```python
from build123d import *

# Parameters (mm, degrees)
SKETCH_1_R               = 2.05
SKETCH_1_R_2             = 1.05
SKETCH_1_R_3             = 1.55
SKETCH_1_R_4             = 1.25
EXTRUDE_1_DEPTH          = 4
EXTRUDE_START            = -4
EXTRUDE_2_DEPTH          = 6
SKETCH_4_R               = 1.05
CUT_EXTRUDE_2_DEPTH      = 11
SKETCH_5_R               = 1.2
CUT_EXTRUDE_3_DEPTH      = 114.5
FILLET_1_R               = 5
SKETCH_6_R               = 2.25
CUT_EXTRUDE_4_DEPTH      = 2.5
CHAMFER_1_SIZE           = 1.5
CUT_EXTRUDE_6_DEPTH      = 1
CUT_EXTRUDE_6_DEPTH_BACK = 11


with BuildPart() as part:
    # 草图1 → 凸台-拉伸1 (new body)
    with BuildSketch(Plane.XY):
        Polygon((20, -62), (5, -62), (5, -54.5), (-5, -54.5), (-5, -62), (-20, -62), (-20, 62), (-5, 62), (-5, 54.5), (5, 54.5), (5, 62), (20, 62), align=None)
        with Locations((10, 58.5)):
            Circle(SKETCH_1_R, mode=Mode.SUBTRACT)
        with Locations((-10, 58.5)):
            Circle(SKETCH_1_R, mode=Mode.SUBTRACT)
        with Locations((10, -58.5)):
            Circle(SKETCH_1_R, mode=Mode.SUBTRACT)
        with Locations((-10, -58.5)):
            Circle(SKETCH_1_R, mode=Mode.SUBTRACT)
        with Locations((-11, 6)):
            Circle(SKETCH_1_R_2, mode=Mode.SUBTRACT)
        with Locations((-11, -6)):
            Circle(SKETCH_1_R_2, mode=Mode.SUBTRACT)
        with Locations((11, -6)):
            Circle(SKETCH_1_R_2, mode=Mode.SUBTRACT)
        with Locations((11, 6)):
            Circle(SKETCH_1_R_2, mode=Mode.SUBTRACT)
        with Locations((-11.2, 0)):
            Circle(SKETCH_1_R_3, mode=Mode.SUBTRACT)
        with Locations((-14.35, -10)):
            Circle(SKETCH_1_R_4, mode=Mode.SUBTRACT)
        with Locations((-14.35, 10)):
            Circle(SKETCH_1_R_4, mode=Mode.SUBTRACT)
        with Locations((14.35, 10)):
            Circle(SKETCH_1_R_4, mode=Mode.SUBTRACT)
        with Locations((14.35, -10)):
            Circle(SKETCH_1_R_4, mode=Mode.SUBTRACT)
    extrude(amount=EXTRUDE_1_DEPTH)

    # 草图3 → 凸台-拉伸2 (add)
    with BuildSketch(Plane.XY.offset(4).offset(EXTRUDE_START)):
        Polygon((-20, 14.55), (20, 14.55), (20, 51.5), (14, 51.5), (14, 17.55), (-14, 17.55), (-14, 51.5), (-20, 51.5), align=None)
        Polygon((14, -17.55), (-14, -17.55), (-14, -51.5), (-20, -51.5), (-20, -14.55), (20, -14.55), (20, -51.5), (14, -51.5), align=None)
    extrude(amount=-EXTRUDE_2_DEPTH)

    # 草图4 → 切除-拉伸2 (cut, through all)
    with BuildSketch(Plane.XY.offset(4)):
        with Locations((-4.25753788, -55.24246212)):
            Circle(SKETCH_4_R)
        with Locations((4.25753788, -55.24246212)):
            Circle(SKETCH_4_R)
        with Locations((4.25753788, 55.24246212)):
            Circle(SKETCH_4_R)
        with Locations((-4.25753788, 55.24246212)):
            Circle(SKETCH_4_R)
    extrude(amount=-CUT_EXTRUDE_2_DEPTH, mode=Mode.SUBTRACT)

    # 草图5 → 切除-拉伸3 (cut, through all)
    with BuildSketch(Plane.XZ.offset(51.5)):
        with Locations((17, -3)):
            Circle(SKETCH_5_R)
        with Locations((-17, -3)):
            Circle(SKETCH_5_R)
    extrude(amount=-CUT_EXTRUDE_3_DEPTH, mode=Mode.SUBTRACT)

    # 圆角1
    fillet_1_edges = [part.edges().sort_by_distance(p)[0] for p in [
        (14, -17.55, -3),
        (-14, -17.55, -3),
        (-14, 17.55, -3),
        (14, 17.55, -3),
    ]]
    fillet(fillet_1_edges, radius=FILLET_1_R)

    # 草图6 → 切除-拉伸4 (cut)
    with BuildSketch(Plane.XY.offset(4)):
        with Locations((-11, -6)):
            Circle(SKETCH_6_R)
        with Locations((-11, 6)):
            Circle(SKETCH_6_R)
        with Locations((11, 6)):
            Circle(SKETCH_6_R)
        with Locations((11, -6)):
            Circle(SKETCH_6_R)
    extrude(amount=-CUT_EXTRUDE_4_DEPTH, mode=Mode.SUBTRACT)

    # 倒角1
    chamfer_1_edges = [part.edges().sort_by_distance(p)[0] for p in [
        (-12.75, 0, 4),
    ]]
    chamfer(chamfer_1_edges, length=CHAMFER_1_SIZE)

    # 草图8 → 切除-拉伸6 (cut, two sides)
    with BuildSketch(Plane.XY.offset(4)) as cut_extrude_6_sk:
        with BuildLine():
            Line((6, -17.55), (-6, -17.55))
            ThreePointArc((-6, -17.55), (-8.121320344, -18.428679656), (-9, -20.55))
            Line((-9, -20.55), (-9, -44.55))
            ThreePointArc((-9, -44.55), (-8.121320344, -46.671320344), (-6, -47.55))
            Line((-6, -47.55), (6, -47.55))
            ThreePointArc((6, -47.55), (8.121320344, -46.671320344), (9, -44.55))
            Line((9, -44.55), (9, -20.55))
            ThreePointArc((9, -20.55), (8.121320344, -18.428679656), (6, -17.55))
        make_face()
        with BuildLine():
            Line((-9, 20.55), (-9, 44.55))
            ThreePointArc((-9, 44.55), (-8.121320344, 46.671320344), (-6, 47.55))
            Line((-6, 47.55), (6, 47.55))
            ThreePointArc((6, 47.55), (8.121320344, 46.671320344), (9, 44.55))
            Line((9, 44.55), (9, 20.55))
            ThreePointArc((9, 20.55), (8.121320344, 18.428679656), (6, 17.55))
            Line((6, 17.55), (-6, 17.55))
            ThreePointArc((-6, 17.55), (-8.121320344, 18.428679656), (-9, 20.55))
        make_face()
    extrude(amount=CUT_EXTRUDE_6_DEPTH, mode=Mode.SUBTRACT)
    extrude(cut_extrude_6_sk.sketch, amount=-CUT_EXTRUDE_6_DEPTH_BACK, mode=Mode.SUBTRACT)


solid = part.part
```
For this review, take the finished solid that the model builds, in its own axes (mm). A direction names the side the tool comes from. Give positions to 0.01 mm unless a question says otherwise; leave off trailing zeros. Write each loop counter-clockwise with the first axis right and the second up, starting at its lowest first coordinate (ties: lowest second). Pieces come first, ordered by that corner, then holes.
Item 1: Take a section at D-D (z = -3). Give the number of separate pieces and of enclosed holes in the cut face, and give its area (3 significant figures).
Item 2: Take a section at B-B (y = -10). Give the boundary of the cut face in (x, z).
Item 3: Take a section at C-C (x = 17). Give the boundary of the cut face in (y, z), and give its area (3 significant figures).
Item 4: Insertion check: P1, Ø4.5, axis at x = 1.5, z = 3, coming from the -Y side; P2, Ø20, axis at x = 3.5, y = 29.5, coming from the -Z side; P3, Ø2.5, axis at x = -11, y = 6, coming from the +Z side. Each pin has a flat end and moves straight along its axis. Give the tip position at first contact, or say it passes through.
Item 5: Take a section at A-A (y = -35.5). Give the boundary of the cut face in (x, z).
Item 6: The part is to be moulded in two halves that separate along X. For faces 5 (the face through (14, -37, -3)), 6 (the face through (0, 0, 0)), say which applies: +X half, -X half, draft (parallel to the pull), parting line (faces both ways), or undercut.
Item 7: Machinability: for faces 1 (the face through (-12.5, 18.98, -3.04)), 2 (the face through (-5, 59, 2)), 3 (the face through (-12, 5, 1.5)), 4 (the face through (0, -17.55, -1)), which of the approach directions +Z, -Z, +X, -X, +Y, -Y give a long, thin tool a straight path to every point of the face, cutting with its end or side? Answer none if there is none.
Item 8: Wall thickness on probe 1 along X at (y, z) = (-44, -0.25); probe 2 along X at (y, z) = (-50, -2); probe 3 along Y at (x, z) = (-14.5, -4.5): over which ranges is each line inside the solid? List them lowest first.
Established:
1. separate pieces: 6
1. enclosed holes: 0
1. area: 722 mm2
2. outline: (-20, 0) - (-15.6, 0) - (-15.6, 4) - (-20, 4) - close; (-13.1, 0) - (13.1, 0) - (13.1, 4) - (-13.1, 4) - close; (15.6, 0) - (20, 0) - (20, 4) - (15.6, 4) - close
3. outline: (-62, 0) - (-51.5, 0) - (-51.5, -1.8) - (-14.55, -1.8) - (-14.55, 0) - (14.55, 0) - (14.55, -1.8) - (51.5, -1.8) - (51.5, 0) - (62, 0) - (62, 4) - (-62, 4) - close; (-51.5, -6) - (-14.55, -6) - (-14.55, -4.2) - (-51.5, -4.2) - close; (14.55, -6) - (51.5, -6) - (51.5, -4.2) - (14.55, -4.2) - close
3. area: 762 mm2
4. P1: stops at y = -54.5
4. P2: stops at z = 0
4. P3: stops at z = 1.5
5. outline: (-20, -6) - (-14, -6) - (-14, 0) - (-9, 0) - (-9, 4) - (-20, 4) - close; (9, 0) - (14, 0) - (14, -6) - (20, -6) - (20, 4) - (9, 4) - close; hole circle Ø2.4 at (-17, -3); hole circle Ø2.4 at (17, -3)
6. face 5: undercut
6. face 6: draft
7. face 1: -Z, +Y
7. face 2: +Z, -Z, +Y
7. face 3: +Z
7. face 4: -Z
8. probe 1: x = -20 to -14, 14 to 20
8. probe 2: x = -20 to -17.66, -16.34 to -14, 14 to 16.34, 17.66 to 20
8. probe 3: y = -51.5 to -14.55, 14.55 to 51.5
